The listing builds one solid part. Answer for the finished solid, in the listing's coordinates (mm). Face numbers are marked on the shaded views. A direction names the side the tool comes from. Give positions to 0.01 mm unless a question says otherwise; leave off trailing zeros. Write each loop counter-clockwise with the first axis right and the second up, starting at its lowest first coordinate (ties: lowest second). Pieces come first, ordered by that corner, then holes. Notation, with made-up numbers: M -37,-39.5 L -14,-39.5 A34 cw -14,-0.5 Z; hole C 32.25,-36 d5. An arc over 180 degrees is marked long. Return JSON: item names as keys, results as strings.
from build123d import *

# Parameters (mm, degrees)
SKETCH1_W                      = 5
SKETCH1_H                      = 140
BOSS_EXTRUDE1_DEPTH            = 100
CUT_EXTRUDE3_DEPTH             = 202.556443707
CUT_EXTRUDE3_DEPTH_BACK        = 202.556443707
SKETCH4_4_R                    = 9.85
CUT_EXTRUDE4_DEPTH             = 3
CUT_EXTRUDE5_START             = 103
SKETCH4_6_R                    = 9.85
CUT_EXTRUDE5_DEPTH             = 103
CUT_EXTRUDE6_REACH             = 206.206
SKETCH5_R                      = 2.25
CUT_EXTRUDE6_DIRECTION_2_DEPTH = 205.205778567
CUT_EXTRUDE7_REACH             = 201.841
SKETCH6_R                      = 2.25
SKETCH7_W                      = 12
SKETCH7_H                      = 15
CUT_EXTRUDE8_DEPTH             = 197.242821038
FILLET3_R                      = 2.5
FILLET4_R                      = 2.5
FILLET5_R                      = 5
FILLET6_R                      = 5


with BuildPart() as part:
    # Sketch1 → Boss-Extrude1 (new body)
    with BuildSketch(Plane.XY):
        with Locations((-13.100610125, 70)):
            Rectangle(SKETCH1_W, SKETCH1_H)
        Polygon((-10.600610125, 0), (-15.600610125, 0), (-15.600610125, -5), (94.399389875, -5), (94.399389875, 0), (89.399389875, 0), align=None)
        with Locations((91.899389875, 70)):
            Rectangle(SKETCH1_W, SKETCH1_H)
    extrude(amount=-BOSS_EXTRUDE1_DEPTH)

    # Sketch4 → Cut-Extrude3 (cut, two sides: drawn at the far end of the back side and taken through both)
    with BuildSketch(Plane.ZY.offset(-89.399389875).offset(-CUT_EXTRUDE3_DEPTH_BACK)):
        with BuildLine():
            ThreePointArc((-89.05, 45), (-82.05, 38), (-75.05, 45))
            Line((-75.05, 45), (-82.05, 45))
            Line((-82.05, 45), (-89.05, 45))
        make_face()
        with BuildLine():
            Line((-82.05, 45), (-75.05, 45))
            ThreePointArc((-75.05, 45), (-82.05, 52), (-89.05, 45))
            Line((-89.05, 45), (-82.05, 45))
        make_face()
        with BuildLine():
            ThreePointArc((-57, 45), (-50, 38), (-43, 45))
            Line((-43, 45), (-50, 45))
            Line((-50, 45), (-57, 45))
        make_face()
        with BuildLine():
            Line((-50, 45), (-43, 45))
            ThreePointArc((-43, 45), (-50, 52), (-57, 45))
            Line((-57, 45), (-50, 45))
        make_face()
        with BuildLine():
            ThreePointArc((-24.95, 45), (-17.95, 38), (-10.95, 45))
            Line((-10.95, 45), (-17.95, 45))
            Line((-17.95, 45), (-24.95, 45))
        make_face()
        with BuildLine():
            Line((-17.95, 45), (-10.95, 45))
            ThreePointArc((-10.95, 45), (-17.95, 52), (-24.95, 45))
            Line((-24.95, 45), (-17.95, 45))
        make_face()
    extrude(amount=CUT_EXTRUDE3_DEPTH + CUT_EXTRUDE3_DEPTH_BACK, mode=Mode.SUBTRACT)

    # Sketch4<4> → Cut-Extrude4 (cut)
    with BuildSketch(Plane.ZY.offset(-89.399389875)):
        with Locations((-50, 45)):
            Circle(SKETCH4_4_R)
        with Locations((-82.05, 45)):
            Circle(SKETCH4_4_R)
        with Locations((-17.95, 45)):
            Circle(SKETCH4_4_R)
    extrude(amount=-CUT_EXTRUDE4_DEPTH, mode=Mode.SUBTRACT)

    # Sketch4<6> → Cut-Extrude5 (cut)
    with BuildSketch(Plane.ZY.offset(-89.399389875).offset(CUT_EXTRUDE5_START)):
        with Locations((-50, 45)):
            Circle(SKETCH4_6_R)
        with Locations((-82.05, 45)):
            Circle(SKETCH4_6_R)
        with Locations((-17.95, 45)):
            Circle(SKETCH4_6_R)
    extrude(amount=-CUT_EXTRUDE5_DEPTH, mode=Mode.SUBTRACT)

    # Sketch5 → Cut-Extrude6 (cut, up to next)
    with BuildSketch(Plane.ZY.offset(15.600610125), mode=Mode.PRIVATE) as cut_extrude6_sk1:
        with Locations(Location((-78.75, 119.5, 0), (0, 0, 90))):
            Circle(SKETCH5_R)
    cut_extrude6_tool1 = extrude(cut_extrude6_sk1.sketch, amount=-CUT_EXTRUDE6_REACH, mode=Mode.PRIVATE) & part.part
    # Sketch5 → Cut-Extrude6 (cut, up to next)
    with BuildSketch(Plane.ZY.offset(15.600610125), mode=Mode.PRIVATE) as cut_extrude6_sk2:
        with Locations(Location((-21.25, 119.5, 0), (0, 0, 90))):
            Circle(SKETCH5_R)
    cut_extrude6_tool2 = extrude(cut_extrude6_sk2.sketch, amount=-CUT_EXTRUDE6_REACH, mode=Mode.PRIVATE) & part.part
    add(cut_extrude6_tool1.solids().sort_by_distance((-15.60061, 119.5, -78.75))[0], mode=Mode.SUBTRACT)
    add(cut_extrude6_tool2.solids().sort_by_distance((-15.60061, 119.5, -21.25))[0], mode=Mode.SUBTRACT)

    # Sketch5 → Cut-Extrude6 direction 2 (cut)
    with BuildSketch(Plane.ZY.offset(15.600610125)):
        with Locations(Location((-78.75, 119.5, 0), (0, 0, 90))):
            Circle(SKETCH5_R)
        with Locations(Location((-21.25, 119.5, 0), (0, 0, 90))):
            Circle(SKETCH5_R)
    extrude(amount=CUT_EXTRUDE6_DIRECTION_2_DEPTH, mode=Mode.SUBTRACT)

    # Sketch6 → Cut-Extrude7 (cut, up to next)
    with BuildSketch(Plane.XZ.offset(5), mode=Mode.PRIVATE) as cut_extrude7_sk1:
        with Locations(Location((71.899389875, -50, 0), (0, 0, 270))):
            Circle(SKETCH6_R)
    cut_extrude7_tool1 = extrude(cut_extrude7_sk1.sketch, amount=-CUT_EXTRUDE7_REACH, mode=Mode.PRIVATE) & part.part
    # Sketch6 → Cut-Extrude7 (cut, up to next)
    with BuildSketch(Plane.XZ.offset(5), mode=Mode.PRIVATE) as cut_extrude7_sk2:
        with Locations(Location((6.899389875, -50, 0), (0, 0, 270))):
            Circle(SKETCH6_R)
    cut_extrude7_tool2 = extrude(cut_extrude7_sk2.sketch, amount=-CUT_EXTRUDE7_REACH, mode=Mode.PRIVATE) & part.part
    add(cut_extrude7_tool1.solids().sort_by_distance((71.89939, -5, -50))[0], mode=Mode.SUBTRACT)
    add(cut_extrude7_tool2.solids().sort_by_distance((6.89939, -5, -50))[0], mode=Mode.SUBTRACT)

    # Sketch7 → Cut-Extrude8 (cut, through all)
    with BuildSketch(Plane(origin=(0, 0, 0), x_dir=(1, 0, 0), z_dir=(0, 1, 0))):
        Polygon((45.399389875, 100), (39.399389875, 100), (33.399389875, 100), (33.399389875, 85), (45.399389875, 85), align=None)
        with Locations((39.399389875, 7.5)):
            Rectangle(SKETCH7_W, SKETCH7_H)
    extrude(amount=-CUT_EXTRUDE8_DEPTH, mode=Mode.SUBTRACT)

    # Fillet3
    fillet3_edges = [part.edges().sort_by_distance(p)[0] for p in [
        (33.399389875, 0, -7.5),
        (33.399389875, -2.5, 0),
        (39.399389875, 0, -15),
        (33.399389875, -2.5, -15),
        (45.399389875, -5, -7.5),
        (45.399389875, -2.5, -15),
        (45.399389875, -2.5, 0),
        (33.399389875, -5, -7.5),
        (39.399389875, -5, -15),
        (45.399389875, 0, -7.5),
    ]]
    fillet(fillet3_edges, radius=FILLET3_R - 0.0001)  # a hair under: the kernel refuses the full size

    # Fillet4
    fillet4_edges = [part.edges().sort_by_distance(p)[0] for p in [
        (45.399389875, 0, -92.5),
        (45.399389875, -2.5, -100),
        (39.399389875, -5, -85),
        (45.399389875, -2.5, -85),
        (33.399389875, -5, -92.5),
        (33.399389875, -2.5, -85),
        (33.399389875, -2.5, -100),
        (45.399389875, -5, -92.5),
        (33.399389875, 0, -92.5),
        (39.399389875, 0, -85),
    ]]
    fillet(fillet4_edges, radius=FILLET4_R - 0.0001)  # a hair under: the kernel refuses the full size

    # Fillet5
    fillet5_edges = [part.edges().sort_by_distance(p)[0] for p in [
        (89.399389875, 0, -50),
        (-10.600610125, 0, -50),
    ]]
    fillet(fillet5_edges, radius=FILLET5_R)

    # Fillet6
    fillet6_edges = [part.edges().sort_by_distance(p)[0] for p in [
        (91.899389875, 140, -100),
        (-13.100610125, 140, -100),
        (-13.100610125, 140, 0),
        (91.899389875, 140, 0),
    ]]
    fillet(fillet6_edges, radius=FILLET6_R)


solid = part.part
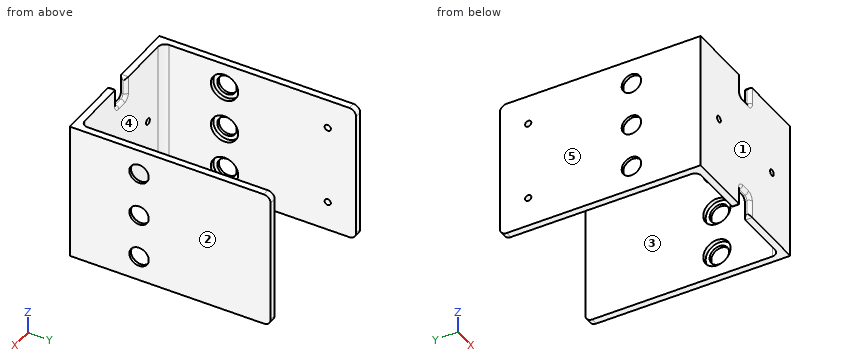
Item 1: Determine the mould class of the marked faces 1, 2 and 3 for opening direction X: +X half, -X half, draft (parallel to the pull), parting line (faces both ways), or undercut.
Geometry results:
{"face 1": "draft", "face 2": "+X half", "face 3": "undercut"}
Item 2: A cutting plane is placed at B-B, the plane z = -50. Count the separate pieces of the cut face and the enclosed holes in it, plus the area to 3 significant figures.
Geometry results:
{"separate pieces": "5", "enclosed holes": "0", "area": "1,740 mm2"}
Item 3: Which of the six approach directions +Z, -Z, +X, -X, +Y, -Y give full straight-line access (tool end or side, diameter ignored) to the marked faces 4 and 5?
Geometry results:
{"face 4": "+Z, -Z, +Y", "face 5": "+Z, -Z, -X, +Y, -Y"}
Item 4: A cutting plane is placed at A-A, the plane y = 25.5. Write down the section's boundary in (x, z), plus the area to 3 significant figures.
Geometry results:
{"outline": "M -15.6,-100 L -10.6,-100 L -10.6,0 L -15.6,0 Z; M 89.4,-100 L 94.4,-100 L 94.4,0 L 89.4,0 Z", "area": "1,000 mm2"}
Item 5: Given pin 1 Ø10 at (x, z) = (7.5, -66.5) entering from +Y; pin 2 Ø3.5 at (x, z) = (71.9, -50) entering from -Y, each flat-ended and moving along its own axis, determine where each tip first touches the part or whether it passes through.
Geometry results:
{"pin 1": "stops at y = 0", "pin 2": "passes through"}
Item 6: A cutting plane is placed at C-C, the plane y = 119.5. Write down the section's boundary in (x, z), plus the area to 3 significant figures.
Geometry results:
{"outline": "M -15.6,-100 L -10.6,-100 L -10.6,-81 L -15.6,-81 Z; M -15.6,-76.5 L -10.6,-76.5 L -10.6,-23.5 L -15.6,-23.5 Z; M -15.6,-19 L -10.6,-19 L -10.6,0 L -15.6,0 Z; M 89.4,-100 L 94.4,-100 L 94.4,0 L 89.4,0 Z", "area": "955 mm2"}
Item 7: Find the intervals of material crossed by line 1 (Z direction, x = -14.9, y = 45); line 2 (X direction, y = 95.5, z = -57); line 3 (Y direction, x = -11.7, z = -17.95), in increasing order.
Geometry results:
{"line 1": "z = -100 to -89.05, -75.05 to -57, -43 to -24.95, -10.95 to 0", "line 2": "x = -15.6 to -10.6, 89.4 to 94.4", "line 3": "y = -5 to 35.15, 54.85 to 140"}
